Check sheet for the modelled part. Datum: model origin and axes. Units: mm. Face numbers are marked on the shaded views. A direction names the side the tool comes from. Round coordinates to 2 decimals unless told otherwise and drop trailing zeros. Order: outer loops, then holes, each group sorted by start corner. A loop starts at its lowest first (then second) coordinate and runs counter-clockwise, first axis right, second up. Notation, with made-up numbers: (88.25, -12) -> (131.25, -12) arc R32 ccw to (131.25, 21) -> close; hole circle Ø5 at (-29.5, 37). An arc over 180 degrees is marked (long way). Use CSV: the item, a comma, the result in double quotes.
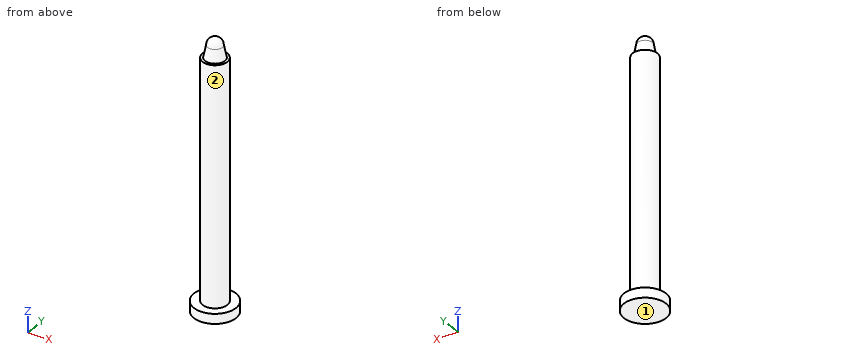
```python
from build123d import *

# Parameters (mm, degrees)
F0_R     = 8.5
F1_DEPTH = 4
F2_R     = 5
F3_DEPTH = 100


with BuildPart() as f1:
    # F0 (on Top) → F1 (new body)
    with BuildSketch(Plane.XY):
        Circle(F0_R)
    extrude(amount=F1_DEPTH)

    # F2 (on Top) → F3 (join)
    with BuildSketch(Plane.XY):
        Circle(F2_R)
    extrude(amount=F3_DEPTH)

    # F4 (on Right) → F5 (revolve)
    with BuildSketch(Plane.YZ):
        Polygon((3, 105), (0, 105), (0, 100), (4, 100), align=None)
    revolve(axis=Axis((0, 0, 102.5), (0, 0, -1)))

    # F6 (on Right) → F7 (revolve)
    with BuildSketch(Plane.YZ):
        with BuildLine():
            ThreePointArc((3, 105), (2.12132, 107.12132), (0, 108))
            Line((0, 108), (0, 105))
            Line((0, 105), (3, 105))
        make_face()
    revolve(axis=Axis((0, 0, 106.5), (0, 0, -1)))


solid = f1.part
```
Q1. Sectioned sample at B-B, the plane z = 48. Enter the section's corners in (x, y).
Result sheet:
outline,"circle Ø10 at (0, 0)"
Q2. Sectioned sample at A-A, the plane x = 7.5. Enter the section's corners in (y, z), then the cut area to 3 significant figures.
Result sheet:
outline,"(-4, 0) -> (4, 0) -> (4, 4) -> (-4, 4) -> close"
area,"32.0 mm^2"
Q3. Go/stop test with flat-tipped pins: pin 1 (10 mm diameter, centred on x = 0, y = -6.5, fed in from +Z); pin 2 (3 mm diameter, centred on x = 1.5, y = -2, fed in from +Z); pin 3 (1 mm diameter, centred on x = 2, y = -1.5, fed in from +Z). Record where each tip stops, or that it passes through.
Result sheet:
pin 1,"stops at z = 107.6"
pin 2,"stops at z = 107.83"
pin 3,"stops at z = 107.24"
Q4. Sectioned sample at C-C, the plane y = -7.25. Enter the section's corners in (x, z), then the cut area to 3 significant figures.
Result sheet:
outline,"(-4.44, 0) -> (4.44, 0) -> (4.44, 4) -> (-4.44, 4) -> close"
area,"35.5 mm^2"
Q5. Access from +Z, -Z, +X, -X, +Y, -Y to the whole of each face (thin tool, end or side, straight path). Record for the marked faces 1 and 2.
Result sheet:
face 1,"-Z, +X, -X, +Y, -Y"
face 2,"+Z"
Q6. Scan lines: L1, parallel to Z at x = 4.5, y = 4.25; L2, parallel to Y at x = 4, z = 89; L3, parallel to Z at x = 3.75, y = -3. Record each from-to range of solid material in increasing order.
Result sheet:
L1,"z = 0 to 4"
L2,"y = -3 to 3"
L3,"z = 0 to 100"
